The model under review builds one solid part; all positions refer to its coordinate system, in mm. A direction names the side the tool comes from. Round coordinates to 2 decimals unless told otherwise and drop trailing zeros. Write each loop counter-clockwise with the first axis right and the second up, starting at its lowest first coordinate (ties: lowest second). Pieces come first, ordered by that corner, then holes. Notation, with made-up numbers: (33, -27.5) -> (37, -27.5) arc R14 cw to (37, -21.5) -> close; hole circle Ø11 at (71, 79.5). An arc over 180 degrees is marked (long way). Use CSV: the item, a comma, the result in double quotes. Start each with the question number.
1) Take a section at C-C, the plane z = 21. Give the boundary of the cut face in (x, y).
2) Machinability: for faces 1 (the face through (-20.689, -3, 10)), 2 (the face through (0, -3, 28.855)), 3 (the face through (14, -5, 0.056)), which of the approach directions +Z, -Z, +X, -X, +Y, -Y give a long, thin tool a straight path to every point of the face, cutting with its end or side? Answer none if there is none.
3) For pin 1 Ø4 at (x, z) = (12, -3.5) entering from -Y, flat-tipped, find the tip position at first contact; note if it passes through.
4) Take a section at A-A, the plane z = 12.5. Give the boundary of the cut face in (x, y).
5) Take a section at D-D, the plane y = -2.5. Give the boundary of the cut face in (x, z).
6) Wall thickness on probe 1 along Z at (x, y) = (4, -4.75); probe 2 along X at (y, z) = (-2.5, 7); probe 3 along X at (y, z) = (-2.75, 13.5): over which ranges is each line inside the solid? List them lowest first. Write a range as [from, to].
7) Take a section at B-B, the plane x = 20. Give the boundary of the cut face in (y, z), then the cut area to 3 significant figures.
from build123d import *

# Parameters (mm, degrees)
F0_W     = 88.9
F0_H     = 44.45
F1_DEPTH = 6.35
F2_W     = 25.4
F2_H     = 12.7
F3_DEPTH = 6.351
F4_W     = 12.7
F4_H     = 7.62
F5_DEPTH = 6.351
F6_W     = 25.4
F6_H     = 12.7
F7_DEPTH = 2.54
F8_W     = 16.51
F8_H     = 7.62
F9_DEPTH = 6.351


with BuildPart() as f1:
    # F0 (on Front) → F1 (new body)
    with BuildSketch(Plane.XZ):
        with Locations((0.276533, 6.62957)):
            Rectangle(F0_W, F0_H)
    extrude(amount=F1_DEPTH)

    # F2 (on face) → F3 (cut, through all)
    with BuildSketch(Plane.XZ.offset(6.35)):
        with Locations((26.547096, 16.865057)):
            Rectangle(F2_W, F2_H)
    extrude(amount=-F3_DEPTH, mode=Mode.SUBTRACT)

    # F4 (on face) → F5 (cut, through all)
    with BuildSketch(Plane.XZ.offset(6.35)):
        with Locations((6.35, 10.021638)):
            Rectangle(F4_W, F4_H)
    extrude(amount=-F5_DEPTH, mode=Mode.SUBTRACT)

    # F6 (on face) → F7 (cut)
    with BuildSketch(Plane.XZ.offset(6.35)):
        with Locations((14.471854, -6.293975)):
            Rectangle(F6_W, F6_H)
    extrude(amount=-F7_DEPTH, mode=Mode.SUBTRACT)

    # F8 (on face) → F9 (cut, through all)
    with BuildSketch(Plane.XZ.offset(6.35)):
        with Locations((-28.943709, 10.228814)):
            Rectangle(F8_W, F8_H)
    extrude(amount=-F9_DEPTH, mode=Mode.SUBTRACT)


solid = f1.part
Values found:
1,outline,"(-44.17, -6.35) -> (13.85, -6.35) -> (13.85, 0) -> (-44.17, 0) -> close; (39.25, -6.35) -> (44.73, -6.35) -> (44.73, 0) -> (39.25, 0) -> close"
2,face 1,"+Y, -Y"
2,face 2,"+Z, +X, -X, +Y, -Y"
2,face 3,"-Y"
3,pin 1,"y = -3.81"
4,outline,"(-44.17, -6.35) -> (-37.2, -6.35) -> (-37.2, 0) -> (-44.17, 0) -> close; (-20.69, -6.35) -> (0, -6.35) -> (0, 0) -> (-20.69, 0) -> close; (12.7, -6.35) -> (13.85, -6.35) -> (13.85, 0) -> (12.7, 0) -> close; (39.25, -6.35) -> (44.73, -6.35) -> (44.73, 0) -> (39.25, 0) -> close"
5,outline,"(-44.17, -15.6) -> (44.73, -15.6) -> (44.73, 28.85) -> (-44.17, 28.85) -> close; hole (-37.2, 6.42) -> (-20.69, 6.42) -> (-20.69, 14.04) -> (-37.2, 14.04) -> close; hole (0, 6.21) -> (12.7, 6.21) -> (12.7, 13.83) -> (0, 13.83) -> close; hole (13.85, 10.52) -> (39.25, 10.52) -> (39.25, 23.22) -> (13.85, 23.22) -> close"
6,probe 1,"[-15.6, -12.64], [0.06, 6.21], [13.83, 28.85]"
6,probe 2,"[-44.17, -37.2], [-20.69, 0], [12.7, 44.73]"
6,probe 3,"[-44.17, -37.2], [-20.69, 0], [12.7, 13.85], [39.25, 44.73]"
7,outline,"(-6.35, -15.6) -> (0, -15.6) -> (0, 10.52) -> (-6.35, 10.52) -> (-6.35, 0.06) -> (-3.81, 0.06) -> (-3.81, -12.64) -> (-6.35, -12.64) -> close; (-6.35, 23.22) -> (0, 23.22) -> (0, 28.85) -> (-6.35, 28.85) -> close"
7,area,"169 mm²"
